```python
from build123d import *

# Parameters (mm, degrees)
BOSS_EXTRUDE2_DEPTH = 28
SKETCH3_W           = 40
SKETCH3_H           = 38
BOSS_EXTRUDE3_DEPTH = 10
CUT_EXTRUDE2_DEPTH  = 8
SKETCH6_W           = 20.7
SKETCH6_H           = 38
CUT_EXTRUDE3_DEPTH  = 43
CUT_EXTRUDE4_DEPTH  = 43
BOSS_EXTRUDE5_DEPTH = 8
SKETCH10_R          = 10
BOSS_EXTRUDE6_DEPTH = 4
SKETCH11_R          = 8
CUT_EXTRUDE5_DEPTH  = 4
SKETCH12_R          = 8
CUT_EXTRUDE6_DEPTH  = 10
SKETCH13_W          = 3.3
SKETCH13_H          = 31.65
CUT_EXTRUDE7_DEPTH  = 10
SKETCH14_W          = 3.3
SKETCH14_H          = 31.65
CUT_EXTRUDE8_DEPTH  = 10
SKETCH15_W          = 16.679991472
SKETCH15_H          = 28
CUT_EXTRUDE9_DEPTH  = 253
SKETCH16_W          = 10.1
SKETCH16_H          = 7
CUT_EXTRUDE11_DEPTH = 13


with BuildPart() as part:
    # Sketch1 → Boss-Extrude2 (new body)
    with BuildSketch(Plane(origin=(0, 0, 0), x_dir=(1, 0, 0), z_dir=(0, 1, 0))):
        Polygon((40, -2), (40, -40), (0, -40), (0, -2), (2.35, -2), (2.35, -2.35), (2.35, -20), (2.35, -37.65), (37.65, -37.65), (37.65, -20), (37.65, -2.35), (37.65, -2), align=None)
    extrude(amount=BOSS_EXTRUDE2_DEPTH)

    # Sketch3 → Boss-Extrude3 (add)
    with BuildSketch(Plane.XZ):
        with Locations((20, 21)):
            Rectangle(SKETCH3_W, SKETCH3_H)
    extrude(amount=BOSS_EXTRUDE3_DEPTH)

    # Sketch5 → Cut-Extrude2 (cut)
    with BuildSketch(Plane(origin=(0, 0, 0), x_dir=(1, 0, 0), z_dir=(0, 1, 0))):
        Polygon((9.65, -20), (9.65, -57.9), (20, -57.9), (30.35, -57.9), (30.35, -20), (30.35, -2), (9.65, -2), align=None)
    extrude(amount=-CUT_EXTRUDE2_DEPTH, mode=Mode.SUBTRACT)

    # Sketch6 → Cut-Extrude3 (cut)
    with BuildSketch(Plane(origin=(0, -8, 0), x_dir=(1, 0, 0), z_dir=(0, 1, 0))):
        with Locations((20, -21)):
            Rectangle(SKETCH6_W, SKETCH6_H)
    extrude(amount=CUT_EXTRUDE3_DEPTH, mode=Mode.SUBTRACT)

    # Sketch7 → Cut-Extrude4 (cut)
    with BuildSketch(Plane(origin=(0, -8, 0), x_dir=(1, 0, 0), z_dir=(0, 1, 0))):
        Polygon((20, -4), (18, -4), (18, -2), (22, -2), (22, -4), align=None)
    extrude(amount=-CUT_EXTRUDE4_DEPTH, mode=Mode.SUBTRACT)

    # Sketch9 → Boss-Extrude5 (add)
    with BuildSketch(Plane.XZ.offset(10)):
        Polygon((30.1, 44.2), (30.1, 40), (32.1, 40), (32.1, 46.2), (18, 46.2), (9.9, 46.2), (7.9, 46.2), (7.9, 40), (9.9, 40), (9.9, 44.2), align=None)
    extrude(amount=-BOSS_EXTRUDE5_DEPTH)

    # Sketch10 → Boss-Extrude6 (add)
    with BuildSketch(Plane.XZ.offset(10)):
        with Locations(Location((20, 20, 0), (0, 0, 270))):
            Circle(SKETCH10_R)
    extrude(amount=BOSS_EXTRUDE6_DEPTH)

    # Sketch11 → Cut-Extrude5 (cut)
    with BuildSketch(Plane(origin=(0, -14, 0), x_dir=(-1, 0, 0), z_dir=(0, -1, 0))):
        with Locations(Location((-20, -20, 0), (0, 0, 90))):
            Circle(SKETCH11_R)
    extrude(amount=-CUT_EXTRUDE5_DEPTH, mode=Mode.SUBTRACT)

    # Sketch12 → Cut-Extrude6 (cut)
    with BuildSketch(Plane.XZ.offset(10)):
        with Locations(Location((20, 20, 0), (0, 0, 270))):
            Circle(SKETCH12_R)
    extrude(amount=-CUT_EXTRUDE6_DEPTH, mode=Mode.SUBTRACT)

    # Sketch13 → Cut-Extrude7 (cut)
    with BuildSketch(Plane(origin=(0, 0, 0), x_dir=(1, 0, 0), z_dir=(0, 1, 0))):
        with Locations((6, -19.825)):
            Rectangle(SKETCH13_W, SKETCH13_H)
    extrude(amount=-CUT_EXTRUDE7_DEPTH, mode=Mode.SUBTRACT)

    # Sketch14 → Cut-Extrude8 (cut)
    with BuildSketch(Plane(origin=(0, 0, 0), x_dir=(1, 0, 0), z_dir=(0, 1, 0))):
        with Locations((34, -19.825)):
            Rectangle(SKETCH14_W, SKETCH14_H)
    extrude(amount=-CUT_EXTRUDE8_DEPTH, mode=Mode.SUBTRACT)

    # Sketch15 → Cut-Extrude9 (cut)
    with BuildSketch(Plane(origin=(40, 0, 0), x_dir=(0, 0, -1), z_dir=(1, 0, 0))):
        with Locations((-21.392853586, 14)):
            Rectangle(SKETCH15_W, SKETCH15_H)
    extrude(amount=-CUT_EXTRUDE9_DEPTH, mode=Mode.SUBTRACT)

    # Sketch16 → Cut-Extrude11 (cut)
    with BuildSketch(Plane.XZ.offset(10)):
        with Locations((20, 36.5)):
            Rectangle(SKETCH16_W, SKETCH16_H)
    extrude(amount=-CUT_EXTRUDE11_DEPTH, mode=Mode.SUBTRACT)


solid = part.part
```
For this review, take the finished solid that the model builds, in its own axes (mm). A direction names the side the tool comes from. Give positions to 0.01 mm unless a question says otherwise; leave off trailing zeros. Order: outer loops, then holes, each group sorted by start corner. A loop starts at its lowest first (then second) coordinate and runs counter-clockwise, first axis right, second up.
1) Take a section at C-C (y = 9). Give the boundary of the cut face in (x, z), then the cut area to 3 significant figures.
2) Take a section at A-A (x = 7). Give the boundary of the cut face in (y, z).
3) Take a section at B-B (z = 20). Give the boundary of the cut face in (x, y).
4) For faces 1 (the face through (18, -9, 3)), 2 (the face through (14.95, -9, 36)), 3 (the face through (2, 28, 37)), 4 (the face through (39, 14, 13.053)), list the 3-axis set-ups (+Z, -Z, +X, -X, +Y, -Y) from which the entire face can be reached by the end or side of a thin tool; tool diameter is ignored.
5) The part is to be moulded in two halves that separate along Z. For faces 5 (the face through (30.35, -1, 25)), 6 (the face through (6, 14, 37.65)), 7 (the face through (39, 14, 29.733)), 8 (the face through (4.35, -5, 20)), say which applies: released by +Z, released by -Z, zero draft, split by the parting line, or undercut.
6) Take a section at D-D (x = 20). Give the boundary of the cut face in (y, z).
7) Wall thickness on line 1 (X direction, y = -7.5, z = 27); line 2 (Z direction, x = 33, y = -4); line 3 (X direction, y = 14.5, z = 11.5): over which ranges is each line inside the solid? List them lowest first.
8) Insertion check: pin 1 (8 mm diameter, centred on x = 31.5, z = 9, fed in from -Y); pin 2 (1.3 mm diameter, centred on y = -6.5, z = 41.5, fed in from -X); pin 3 (3.5 mm diameter, centred on x = 6, y = 9, fed in from -Z); pin 4 (2 mm diameter, centred on y = 12.5, z = 14.5, fed in from +X). Each pin has a flat end and moves straight along its axis. Give the tip position at first contact, or say it passes through.
Derived:
1. outline: (0, 2) - (2.35, 2) - (2.35, 13.05) - (0, 13.05) - close; (0, 29.73) - (2.35, 29.73) - (2.35, 37.65) - (9.65, 37.65) - (9.65, 40) - (0, 40) - close; (30.35, 37.65) - (37.65, 37.65) - (37.65, 29.73) - (40, 29.73) - (40, 40) - (30.35, 40) - close; (37.65, 2) - (40, 2) - (40, 13.05) - (37.65, 13.05) - close
1. area: 135 mm2
2. outline: (-10, 2) - (0, 2) - (0, 4) - (-10, 4) - close; (-10, 35.65) - (0, 35.65) - (0, 37.65) - (28, 37.65) - (28, 40) - (-10, 40) - close
3. outline: (0, -10) - (4.35, -10) - (4.35, 0) - (0, 0) - close; (7.65, -10) - (10, -10) - (10, -14) - (12, -14) - (12, -8) - (9.65, -8) - (9.65, 0) - (7.65, 0) - close; (28, -14) - (30, -14) - (30, -10) - (32.35, -10) - (32.35, 0) - (30.35, 0) - (30.35, -8) - (28, -8) - close; (35.65, -10) - (40, -10) - (40, 0) - (35.65, 0) - close
4. face 1: -Z, +Y, -Y
4. face 2: +Y, -Y
4. face 3: +Z, -Z, +X, -X, +Y
4. face 4: +X, -X, +Y
5. face 5: zero draft
5. face 6: released by -Z
5. face 7: undercut
5. face 8: undercut
6. outline: (-14, 10) - (-10, 10) - (-10, 4) - (-8, 4) - (-8, 12) - (-14, 12) - close; (-14, 28) - (-8, 28) - (-8, 33) - (-10, 33) - (-10, 30) - (-14, 30) - close; (-10, 44.2) - (-2, 44.2) - (-2, 46.2) - (-10, 46.2) - close
7. line 1: x = 0 to 4.35, 7.65 to 9.65, 30.35 to 32.35, 35.65 to 40
7. line 2: z = 2 to 4, 35.65 to 40
7. line 3: x = 0 to 2.35, 37.65 to 40
8. pin 1: stops at y = -10
8. pin 2: stops at x = 7.9
8. pin 3: stops at z = 37.65
8. pin 4: passes through
